Study the drawing (mm; zero at the part's minimum x, y, z) and answer. A direction names the side the tool comes from. Give positions to 0.01 mm unless a question says otherwise; leave off trailing zeros. Loops run counter-clockwise (first coordinate to the right, second up) from the corner with the lowest first, then second, coordinate; pieces in that order, holes last. Notation, with made-up numbers: (67, 78) -> (92, 78) arc R22 cw to (92, 89) -> close; hole circle Ø2 at (7.25, -36.5). An arc over 180 degrees is marked (long way). One line per question, with ' | ' between items. Start each with the question number.
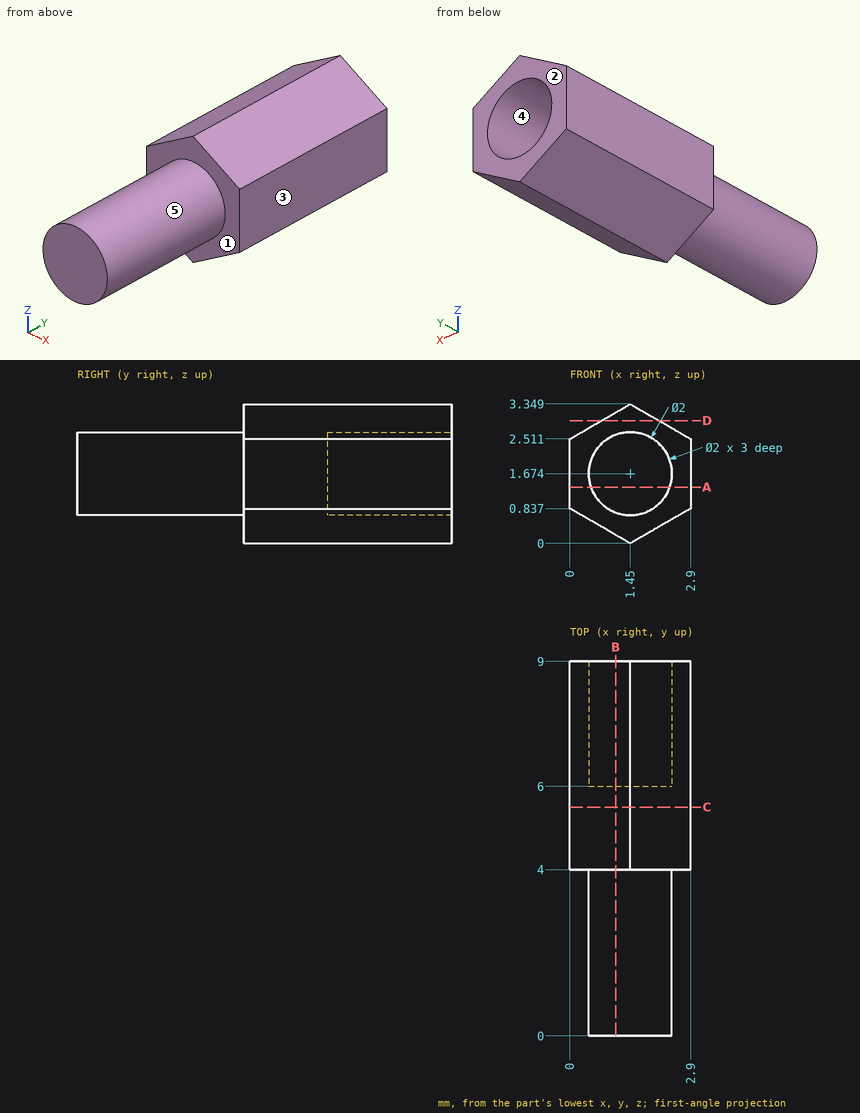
1. The part is cut by section A-A (z = 1.35). Write down the section's boundary in (x, y) (1 decimal).
2. The part is cut by section D-D (z = 2.95). Write down the section's boundary in (x, y).
3. Determine the mould class of the marked faces 3, 4 and 5 for opening direction X: released by +X, released by -X, zero draft, split by the parting line, or undercut.
4. For the marked faces 1 and 2, determine the directions among +Z, -Z, +X, -X, +Y, -Y from which every point of the face is accessible in a straight line to the end or side of a thin tool.
5. This flat-tipped pin is pushed along its axis until it touches: pin 1 Ø1.5 at (x, y) = (1, 3) entering from -Z. Where does it stop, or does it pass through?
6. Straight lines are drawn through the part: L1, parallel to Z at x = 1.8, y = 8 (1 decimal); L2, parallel to Y at x = 2.1, z = 0.7; L3, parallel to Y at x = 1.9, z = 1.35. For each, find the intervals that lie inside material, in ascending order.
7. The part is cut by section C-C (y = 5.5). Write down the section's boundary in (x, z).
8. The part is cut by section B-B (x = 1.1). Write down the section's boundary in (y, z), plus the area to 3 significant figures.
Check sheet entries:
1) outline: (0, 4) -> (0.5, 4) -> (0.5, 0) -> (2.4, 0) -> (2.4, 4) -> (2.9, 4) -> (2.9, 9) -> (2.4, 9) -> (2.4, 6) -> (0.5, 6) -> (0.5, 9) -> (0, 9) -> close
2) outline: (0.76, 4) -> (2.14, 4) -> (2.14, 9) -> (0.76, 9) -> close
3) face 3: released by +X | face 4: undercut | face 5: split by the parting line
4) face 1: -Y | face 2: +Z, -Z, +X, -X, +Y
5) pin 1: stops at z = 0.67
6) L1: z = 0.2 to 0.7, 2.6 to 3.1 | L2: y = 4 to 9 | L3: y = 0 to 6
7) outline: (0, 0.84) -> (1.45, 0) -> (2.9, 0.84) -> (2.9, 2.51) -> (1.45, 3.35) -> (0, 2.51) -> close
8) outline: (0, 0.74) -> (4, 0.74) -> (4, 0.2) -> (9, 0.2) -> (9, 0.74) -> (6, 0.74) -> (6, 2.61) -> (9, 2.61) -> (9, 3.15) -> (4, 3.15) -> (4, 2.61) -> (0, 2.61) -> close | area: 16.6 mm^2
